Part model, mm, in its own coordinate system. A direction names the side the tool comes from. Give positions to 0.01 mm unless a question says otherwise; leave off trailing zeros. Write each loop counter-clockwise with the first axis right and the second up, starting at its lowest first coordinate (ties: lowest second). Pieces come first, ordered by that corner, then holes.
Autodesk Inventor part; units mm, degrees
ref_plane "Work Plane1" through (14.605, 0, 0) normal (0, 0, -1) x (1, 0, 0)
ref_plane "YZ Plane" through (0, 0, 0) normal (1, 0, 0) x (0, 1, 0)
ref_plane "XZ Plane" through (0, 0, 0) normal (0, 1, 0) x (-1, 0, 0)
sketch "Sketch1" plane through (0, 0, 0) normal (0, 0, 1) x (1, 0, 0)
  line L0 (0, 1.4224) -> (0, 0)
  line L1 (3.81, 1.4224) -> (25.4, 1.4224)
  line L2 (25.4, 1.4224) -> (25.4, 0)
  line L3 (25.4, 0) -> (0, 0)
  line L4 (3.81, 1.4224) -> (3.4925, 1.4224)
  line L5 (3.4925, 1.4224) -> (0, 1.4224)
  line L6 (-5.08, 0) -> (30.48, 0)
  line L7 (0, -0.2845) -> (0, 1.7069)
  dimension "d0" = 25.4
  dimension "d1" = 21.59
  dimension "d2" = 2.8448
  dimension "d13" = 0.3175
  dimension "d24" = 2.8448
revolve "Body" add sketch "Sketch1" angle 360 about axis through (25.4, 0, 0) along (-1, 0, 0)
sketch "Sketch2" plane through (0, 0, 0) normal (-1, 0, 0) x (0, 0, 1)
  line L0 (0, 3.2116) -> (2.7813, 1.6058)
  line L1 (2.7813, 1.6058) -> (2.7813, -1.6058)
  line L2 (2.7813, -1.6058) -> (0, -3.2116)
  line L3 (0, -3.2116) -> (-2.7813, -1.6058)
  line L4 (-2.7813, -1.6058) -> (-2.7813, 1.6058)
  line L5 (-2.7813, 1.6058) -> (0, 3.2116)
  circle A0 centre (0, 0) radius 1.4224
  dimension "d8" = 5.5626
extrude "Head" add sketch "Sketch2" along normal blind 1.524 contours L0 L1 L2 L3 L4 L5 | A0
sketch "Sketch3" plane through (-1.524, 0, 0) normal (-1, 0, 0) x (0, 0, 1)
  circle A0 centre (0, 0) radius 2.225
  point P0 (0, 0)
  dimension "d17" = 4.4501
extrude "Indent" cut sketch "Sketch3" against normal blind 0.1524
sketch "Sketch4" plane through (0, 0, 0) normal (0, 0, 1) x (1, 0, 0)
  line L0 (-1.524, 0.4953) -> (-0.6095, 0.4953)
  line L1 (-0.6095, 0.4953) -> (-0.6095, -0.4953)
  line L2 (-0.6095, -0.4953) -> (-1.524, -0.4953)
  line L3 (-1.524, -0.4953) -> (-1.524, 0.4953)
  line L4 (-0.6095, 0) -> (-1.524, 0) construction
  line L5 (-1.7069, 0) -> (-0.4266, 0)
  line L6 (-1.524, 1.6058) -> (-1.524, -1.6058)
  dimension "d9" = 0.9906
  dimension "d10" = 0.9145
extrude "Slot" cut sketch "Sketch4" along normal through all both and the other way through all
sketch "Sketch5" plane through (0, 0, 0) normal (0, 0, 1) x (1, 0, 0)
  line L0 (-1.8288, 0) -> (0.3048, 0)
  line L1 (-1.524, 3.2116) -> (-1.524, 2.7813)
  line L2 (-1.524, 2.7813) -> (-1.2756, 3.2116)
  line L3 (-1.2756, 3.2116) -> (-1.524, 3.2116)
  line L4 (0, 3.2116) -> (-1.524, 3.2116)
  line L5 (-1.524, 3.2116) -> (-1.524, 1.6058)
  dimension "d22" = 30
  dimension "d23" = 5.5626
revolve "Chamfer1" cut sketch "Sketch5" angle 360 about axis through (-10, 0, 0) along (1, 0, 0)
fillet "Fillet1" radius 0.0284 1 edges at (0, -1.4224, 0)
thread "Thread"
chamfer "Chamfer2" distance 0.3175 distance2 0.3175 1 edges at (25.4, -1.4224, 0) measured on face at (25.4, -0.5703, -0.3902)
ref_plane "Work Plane1" through (14.605, 0, 0) normal (0, 0, -1) x (1, 0, 0)
equation "\"d0\" = NLG"
equation "\"d1\" = GEL"
equation "\"d2\" = GD"
equation "\"d13\" = GAL"
equation "\"d24\" = BDM"
equation "\"d8\" = SW"
equation "\"d3\" = KOH - SD"
equation "\"d17\" = KOD2"
equation "\"d18\" = KOH2"
equation "\"d9\" = SBR"
equation "\"d22\" = ANG1"
equation "\"d23\" = SW"
equation "\"d16\" = RR"
equation "\"d14\" = GEL"
equation "\"d5\" = -0.5 * SPD + 0.5 * GD"
equation "\"d6\" = GUL"
equation "\"NLG\" = 25.4"
equation "\"GD\" = NND"
equation "\"BDM\" = NND"
equation "\"KOH\" = 1.524"
equation "\"GEL\" = 21.59"
equation "\"SW\" = 5.5626"
equation "\"SPD\" = GD1"
equation "\"SD\" = 0"
equation "\"ANG1\" = 30deg"
equation "\"GAL\" = 0.3175"
equation "\"GUL\" = GAL"
equation "\"STI\" = 0.9144"
equation "\"SBR\" = 0.9906"
equation "\"RR\" = 0.02845"
equation "\"KOD2\" = 0.8 * SW"
equation "\"KOH2\" = 0.1 * KOH"
equation "\"SW0\" = SW"
equation "\"THREADDIA\" = 2.8448"
equation "\"SDH\" = SW"
equation "\"E0\" = 1.155 * SW"
equation "\"TOA\" = 30deg"
equation "\"NND\" = 2.8448"
equation "\"GD1\" = 2.2098"
equation "\"SD2\" = NND"
properties part number "ANSI B18.6.3 - 4-40 UNC - 1, SILHHMSI" material "Steel, Mild"
1) Flat gauge pins, fed straight in: P1, Ø3, axis at x = 21, z = -2, coming from the -Y side; P2, Ø0.5, axis at x = -1, z = 1, coming from the -Y side; P3, Ø2, axis at x = 19, y = 0, coming from the -Z side. Where does each tip first touch, or does it go through?
Check result:
P1: stops at y = -1.33
P2: stops at y = -2.78
P3: stops at z = -1.42
2) Drill centre lines: L1, parallel to X at y = 0.75, z = -1.75; L2, parallel to X at y = -2.25, z = -0.85; L3, parallel to Y at x = 11, z = 0.05. Where is each one in solid material? Low to high.
Check result:
L1: x = -1.37 to 0
L2: x = -1.52 to 0
L3: y = -1.42 to 1.42
3) Mould opens along Y. For faces 1 (the flat face through (-0.4, 0, 2.781)), 2 (the flat face through (-0.75, -2.42, -1.37)), 3 (the flat face through (-0.61, 0, 0)) say: +Y half, -Y half, draft (parallel to the pull), parting line (faces both ways), or undercut.
Check result:
face 1: draft
face 2: -Y half
face 3: undercut
4) 3-axis set-ups, long thin cutter, end or side, ignore diameter. For faces 4 (the flat face through (-1.372, -1, 0)), 5 (the flat face through (0, 1.5, -0.7)), 6 (the flat face through (-1, 0.495, 0)): which of +Z, -Z, +X, -X, +Y, -Y reach the whole face in a straight line?
Check result:
face 4: -X
face 5: +X
face 6: +Z, -Z, -X
5) Saw through at A-A (y = 0). Write the cut outline in (x, z).
Check result:
outline: (-0.61, -2.78) - (0, -2.78) - (0, -1.45) arc R0.03 cw to (0.03, -1.42) - (25.08, -1.42) - (25.4, -1.1) - (25.4, 1.1) - (25.08, 1.42) - (0.03, 1.42) arc R0.03 cw to (0, 1.45) - (0, 2.78) - (-0.61, 2.78) - close
6) Saw through at B-B (x = 16). Write the cut outline in (y, z), and give its area (3 significant figures).
Check result:
outline: circle Ø2.84 at (0, 0)
area: 6.36 mm2
